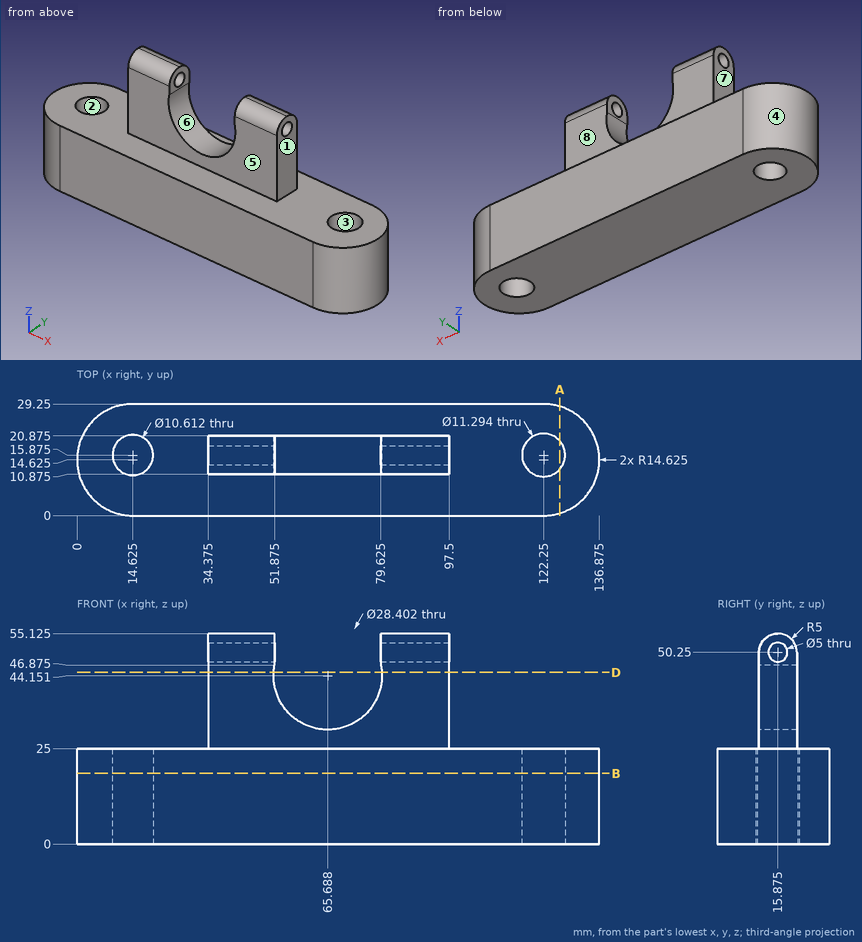
Geometry check sheet. Reference: drawing and pictorial views, mm from the part's lowest x, y, z. A direction names the side the tool comes from. Give positions to 0.01 mm unless a question says otherwise; leave off trailing zeros. Loops run counter-clockwise (first coordinate to the right, second up) from the corner with the lowest first, then second, coordinate; pieces in that order, holes last. Notation, with made-up numbers: (34, 26) - (42, 26) arc R26 cw to (42, 51) - close; hole circle Ø3 at (-17.75, -8). An arc over 180 degrees is marked (long way). Use CSV: the item, a comma, the result in double quotes. Start each with the question number.
Q1. Section check D-D, the plane z = 45. Record the cut outline in (x, y) (1 decimal), and give its area (3 significant figures).
Q2. Section check A-A, the plane x = 126.5. Record the cut outline in (y, z).
Q3. Scan lines: probe 1 along Z at (x, y) = (82, 16.25); probe 2 along X at (y, z) = (18.75, 22) (1 decimal); probe 3 along Z at (x, y) = (22, 5.75). Record each from-to range of solid material in increasing order. Write a range as from..to.
Q4. Release check for a two-part mould opening along X. For the marked faces 1, 2, 3 and 4 record: +X half, -X half, draft (parallel to the pull), parting line (faces both ways), or undercut.
Q5. Section check B-B, the plane z = 18.5. Count the separate pieces of the cut face and the enclosed holes in it, and give its area (3 significant figures).
Q6. Access from +Z, -Z, +X, -X, +Y, -Y to the whole of each face (thin tool, end or side, straight path). Record for the marked faces 5, 6, 7 and 8.
Q7. Go/stop test with flat-tipped pins: pin 1 Ø6.5 at (x, y) = (14.625, 15.875) entering from -Z; pin 2 Ø8 at (x, z) = (83.5, 30) entering from -Y (1 decimal); pin 3 Ø6.5 at (y, z) = (15.88, 50.25) entering from -X (1 decimal); pin 4 Ø12 at (y, z) = (24, 21) entering from +X. Record where each tip stops, or that it passes through.
Findings below:
1,outline,"(34.4, 10.9) - (51.5, 10.9) - (51.5, 20.9) - (34.4, 20.9) - close; (79.9, 10.9) - (97.5, 10.9) - (97.5, 20.9) - (79.9, 20.9) - close"
1,area,"348 mm^2"
2,outline,"(0.63, 0) - (12.16, 0) - (12.16, 25) - (0.63, 25) - close; (19.59, 0) - (28.62, 0) - (28.62, 25) - (19.59, 25) - close"
3,probe 1,"z = 0..47.78, 52.72..55.11"
3,probe 2,"x = 0.6..10.2, 19.1..117.4, 127.1..136.3"
3,probe 3,"z = 0..25"
4,face 1,"+X half"
4,face 2,"undercut"
4,face 3,"undercut"
4,face 4,"-X half"
5,separate pieces,"1"
5,enclosed holes,"2"
5,area,"3,630 mm^2"
6,face 5,"+Z, +X, -X, -Y"
6,face 6,"+Y, -Y"
6,face 7,"+Z, -X, +Y, -Y"
6,face 8,"+Z, +X, -X, +Y"
7,pin 1,"passes through"
7,pin 2,"stops at y = 10.9"
7,pin 3,"stops at x = 34.4"
7,pin 4,"stops at x = 136.48"
